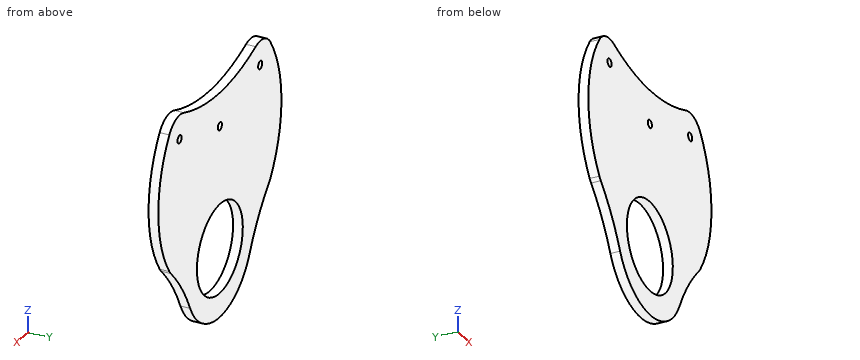
```python
from build123d import *

# Parameters (mm, degrees)
BOSS_EXTRUDE1_DEPTH = 3
SKETCH2_R           = 1.25
SKETCH2_R_2         = 13.875
CUT_EXTRUDE1_DEPTH  = 56.828571826


with BuildPart() as part:
    # Sketch1 → Boss-Extrude1 (new body)
    with BuildSketch(Plane(origin=(0, 0, 0), x_dir=(1, 0, 0), z_dir=(0, 1, 0))):
        with BuildLine():
            ThreePointArc((-30.534150334, -38.289553671), (-37.223372122, -17), (-30.534150334, 4.289553671))
            ThreePointArc((-30.534150334, 4.289553671), (-30.127865646, 4.820197467), (-29.675955722, 5.312566746))
            ThreePointArc((-29.675955722, 5.312566746), (-23.149545378, 13.015308608), (-18.007026439, 21.703275178))
            ThreePointArc((-18.007026439, 21.703275178), (0, 33), (18.007026439, 21.703275178))
            ThreePointArc((18.007026439, 21.703275178), (23.149545378, 13.015308608), (29.675955722, 5.312566746))
            ThreePointArc((29.675955722, 5.312566746), (30.127865646, 4.820197467), (30.534150334, 4.289553671))
            ThreePointArc((30.534150334, 4.289553671), (37.223372122, -17), (30.534150334, -38.289553671))
            ThreePointArc((30.534150334, -38.289553671), (26.570942981, -41.173440783), (21.67283286, -40.993622447))
            ThreePointArc((21.67283286, -40.993622447), (0, -36.942602025), (-21.67283286, -40.993622447))
            ThreePointArc((-21.67283286, -40.993622447), (-26.570942981, -41.173440783), (-30.534150334, -38.289553671))
        make_face()
    extrude(amount=BOSS_EXTRUDE1_DEPTH)

    # Sketch2 → Cut-Extrude1 (cut, through all)
    with BuildSketch(Plane(origin=(0, 3, 0), x_dir=(1, 0, 0), z_dir=(0, 1, 0))):
        with Locations(Location((-24.381936968, -34, 0), (0, 0, 270))):
            Circle(SKETCH2_R)
        with Locations(Location((24.381936968, -34, 0), (0, 0, 270))):
            Circle(SKETCH2_R)
        with Locations(Location((0, -26.5, 0), (0, 0, 270))):
            Circle(SKETCH2_R)
        with Locations(Location((0, 11.63, 0), (0, 0, 270))):
            Circle(SKETCH2_R_2)
    extrude(amount=-CUT_EXTRUDE1_DEPTH, mode=Mode.SUBTRACT)


solid = part.part
```
Can you work these out from the model? Positions are in its coordinate system, mm. Coordinates: 2 decimals unless noted, no trailing zeros. Loops run counter-clockwise (first coordinate to the right, second up) from the corner with the lowest first, then second, coordinate; pieces in that order, holes last. Notation, with made-up numbers: (-31, 80) -> (-4, 80) arc R21 ccw to (-4, 91) -> close; hole circle Ø1 at (57, -2.5). An arc over 180 degrees is marked (long way). Answer as a JSON object with one key per item and string values.
1) For P1, Ø3, axis at x = -0.5, z = 0.5, coming from the -Y side; P2, Ø1.5, axis at y = 2.5, z = -10, coming from the -X side; P3, Ø4, axis at x = 22, z = 15, coming from the -Y side; P4, Ø1, axis at x = -10, y = 1.5, coming from the -Z side, each with a flat end and sliding along its axis, tell me the tip position at first contact or that it passes through.
Results:
{"P1": "passes through", "P2": "stops at x = -26.06", "P3": "stops at y = 0", "P4": "stops at z = -30.6"}
2) If I drill on line 1 (X direction, y = 0.85, z = 34); line 2 (Z direction, x = 0.5, y = 1.3); line 3 (X direction, y = 0.55, z = 18), over which ranges is the centre line in solid material (lowest first)?
Results:
{"line 1": "x = -33.11 to -25.63, -23.13 to 23.13, 25.63 to 33.11", "line 2": "z = -32.99 to -25.5, 2.24 to 25.35, 27.65 to 36.94", "line 3": "x = -37.21 to 37.21"}
3) Imagine slicing it at A-A (x = 0). Please give me the cut outline in (y, z) (3 decimals), then the cut area to 3 significant figures.
Results:
{"outline": "(0, -33) -> (3, -33) -> (3, -25.505) -> (0, -25.505) -> close; (0, 2.245) -> (3, 2.245) -> (3, 25.25) -> (0, 25.25) -> close; (0, 27.75) -> (3, 27.75) -> (3, 36.943) -> (0, 36.943) -> close", "area": "119 mm^2"}
4) Imagine slicing it at C-C (z = 34). Please give me the cut outline in (x, y).
Results:
{"outline": "(-33.11, 0) -> (-25.63, 0) -> (-25.63, 3) -> (-33.11, 3) -> close; (-23.13, 0) -> (23.13, 0) -> (23.13, 3) -> (-23.13, 3) -> close; (25.63, 0) -> (33.11, 0) -> (33.11, 3) -> (25.63, 3) -> close"}
5) Imagine slicing it at D-D (y = 1.85). Please give me the cut outline in (x, z) (3 decimals), then the cut area to 3 significant figures.
Results:
{"outline": "(-30.534, -4.29) arc R7.5 ccw to (-29.676, -5.313) arc R60 cw to (-18.007, -21.703) arc R20 ccw to (18.007, -21.703) arc R60 cw to (29.676, -5.313) arc R7.5 ccw to (30.534, -4.29) arc R37.223 ccw to (30.534, 38.29) arc R7.5 ccw to (21.673, 40.994) arc R60 cw to (-21.673, 40.994) arc R7.5 ccw to (-30.534, 38.29) arc R37.223 ccw to start; hole circle Ø2.5 at (-24.382, 34); hole circle Ø27.75 at (0, -11.63); hole circle Ø2.5 at (0, 26.5); hole circle Ø2.5 at (24.382, 34)", "area": "3,520 mm^2"}
6) Imagine slicing it at B-B (z = -11.63). Please give me the cut outline in (x, y) (3 decimals), then the cut area to 3 significant figures.
Results:
{"outline": "(-24.166, 0) -> (-13.875, 0) -> (-13.875, 3) -> (-24.166, 3) -> close; (13.875, 0) -> (24.166, 0) -> (24.166, 3) -> (13.875, 3) -> close", "area": "61.7 mm^2"}
